Input: part model. Units: mm. Frame: model coordinates. Face numbers are marked on the shaded views. A direction names the side the tool comes from. Give positions to 0.01 mm unless a question says otherwise; leave off trailing zeros. Write each loop counter-clockwise with the first axis right and the second up, starting at its lowest first coordinate (ties: lowest second). Pieces come first, ordered by that corner, then holes. Notation, with made-up numbers: (41.5, -6) -> (54.5, -6) arc R24 cw to (54.5, 24) -> close; hole circle Ø1 at (-30.5, 35). An arc over 180 degrees is marked (long way). Answer as a JSON object with one key per item and string values. Group by question number.
from build123d import *

# Parameters (mm, degrees)
SKETCH1_R                = 6.45
BOSS_EXTRUDE1_DEPTH      = 6.35
FILLET1_R                = 2
SKETCH3_R                = 7.95
SKETCH3_R_2              = 6.45
BOSS_EXTRUDE3_DEPTH      = 3
BOSS_EXTRUDE3_DEPTH_BACK = 15.7
BOSS_EXTRUDE4_DEPTH      = 2
BOSS_EXTRUDE5_DEPTH      = 2
BOSS_EXTRUDE6_DEPTH      = 8.7


with BuildPart() as part:
    # Sketch1 → Boss-Extrude1 (new body, symmetric)
    with BuildSketch(Plane(origin=(0, 0, 0), x_dir=(1, 0, 0), z_dir=(0, 1, 0))):
        Polygon((0, -15.9), (13.76980392, 7.95), (-13.76980392, 7.95), align=None)
        with Locations(Location((0, 0, 0), (0, 0, 270))):  # turned: the seam where the file's is
            Circle(SKETCH1_R, mode=Mode.SUBTRACT)
    extrude(amount=BOSS_EXTRUDE1_DEPTH, both=True)

    # Fillet1
    fillet1_edges = [part.edges().sort_by_distance(p)[0] for p in [
        (-13.76980392, 0, -7.95),
        (13.76980392, 0, -7.95),
        (0, 0, 15.9),
    ]]
    fillet(fillet1_edges, radius=FILLET1_R)

    # Sketch3 → Boss-Extrude3 (add, two sides)
    with BuildSketch(Plane(origin=(0, 6.35, 0), x_dir=(1, 0, 0), z_dir=(0, 1, 0))) as boss_extrude3_sk:
        with Locations(Location((0, 0, 0), (0, 0, 270))):  # turned: the seam where the file's is
            Circle(SKETCH3_R)
        with Locations(Location((0, 0, 0), (0, 0, 270))):  # turned: the seam where the file's is
            Circle(SKETCH3_R_2, mode=Mode.SUBTRACT)
    extrude(amount=BOSS_EXTRUDE3_DEPTH)
    extrude(boss_extrude3_sk.sketch, amount=-BOSS_EXTRUDE3_DEPTH_BACK)

    # Sketch4 → Boss-Extrude4 (add)
    with BuildSketch(Plane(origin=(0, 6.35, 0), x_dir=(1, 0, 0), z_dir=(0, 1, 0))):
        with BuildLine():
            Line((8.183940066, -4.725), (13.336791218, 4.2))
            ThreePointArc((13.336791218, 4.2), (13.336791218, 7.7), (10.305702305, 9.45))
            Line((10.305702305, 9.45), (0, 9.45))
            Line((0, 9.45), (-10.305702305, 9.45))
            ThreePointArc((-10.305702305, 9.45), (-13.336791218, 7.7), (-13.336791218, 4.2))
            Line((-13.336791218, 4.2), (-8.183940066, -4.725))
            Line((-8.183940066, -4.725), (-3.031088913, -13.65))
            ThreePointArc((-3.031088913, -13.65), (0, -15.4), (3.031088913, -13.65))
            Line((3.031088913, -13.65), (8.183940066, -4.725))
        make_face()
        with BuildLine():
            Line((6.88490196, -3.975), (12.037753113, 4.95))
            ThreePointArc((12.037753113, 4.95), (12.037753113, 6.95), (10.305702305, 7.95))
            Line((10.305702305, 7.95), (0, 7.95))
            Line((0, 7.95), (-10.305702305, 7.95))
            ThreePointArc((-10.305702305, 7.95), (-12.037753113, 6.95), (-12.037753113, 4.95))
            Line((-12.037753113, 4.95), (-6.88490196, -3.975))
            Line((-6.88490196, -3.975), (-1.732050808, -12.9))
            ThreePointArc((-1.732050808, -12.9), (0, -13.9), (1.732050808, -12.9))
            Line((1.732050808, -12.9), (6.88490196, -3.975))
        make_face(mode=Mode.SUBTRACT)
    extrude(amount=-BOSS_EXTRUDE4_DEPTH)

    # Sketch5 → Boss-Extrude5 (add)
    with BuildSketch(Plane.XZ.offset(6.35)):
        with BuildLine():
            Line((13.336791218, -4.2), (3.031088913, 13.65))
            ThreePointArc((3.031088913, 13.65), (0, 15.4), (-3.031088913, 13.65))
            Line((-3.031088913, 13.65), (-13.336791218, -4.2))
            ThreePointArc((-13.336791218, -4.2), (-13.336791218, -7.7), (-10.305702305, -9.45))
            Line((-10.305702305, -9.45), (10.305702305, -9.45))
            ThreePointArc((10.305702305, -9.45), (13.336791218, -7.7), (13.336791218, -4.2))
        make_face()
        with BuildLine():
            Line((10.305702305, -7.95), (-10.305702305, -7.95))
            ThreePointArc((-10.305702305, -7.95), (-12.037753113, -6.95), (-12.037753113, -4.95))
            Line((-12.037753113, -4.95), (-1.732050808, 12.9))
            ThreePointArc((-1.732050808, 12.9), (0, 13.9), (1.732050808, 12.9))
            Line((1.732050808, 12.9), (12.037753113, -4.95))
            ThreePointArc((12.037753113, -4.95), (12.037753113, -6.95), (10.305702305, -7.95))
        make_face(mode=Mode.SUBTRACT)
    extrude(amount=-BOSS_EXTRUDE5_DEPTH)

    # Sketch6 → Boss-Extrude6 (add)
    with BuildSketch(Plane.XZ.offset(-4.35)):
        with BuildLine():
            Line((-2.165063509, 13.15), (-3.031088913, 13.65))
            ThreePointArc((-3.031088913, 13.65), (0, 15.4), (3.031088913, 13.65))
            Line((3.031088913, 13.65), (2.165063509, 13.15))
            ThreePointArc((2.165063509, 13.15), (1.864007283, 13.565976245), (1.484313483, 13.911669328))
            Line((1.484313483, 13.911669328), (1, 13.632050808))
            ThreePointArc((1, 13.632050808), (0, 13.9), (-1, 13.632050808))
            Line((-1, 13.632050808), (-1.484313483, 13.911669328))
            ThreePointArc((-1.484313483, 13.911669328), (-1.864007283, 13.565976245), (-2.165063509, 13.15))
        make_face()
    extrude(amount=BOSS_EXTRUDE6_DEPTH)


solid = part.part
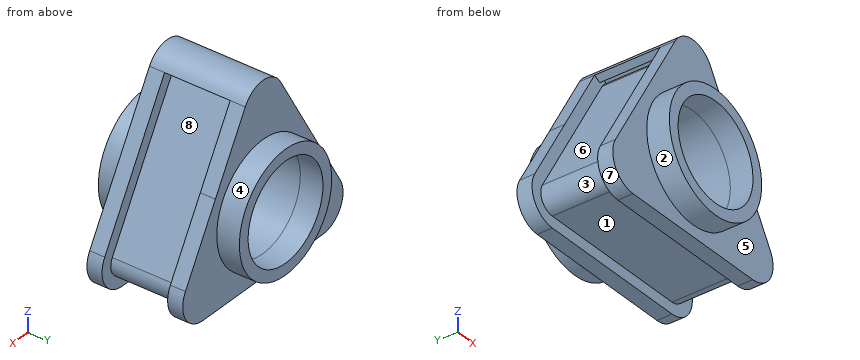
1. Section B-B (y = -2.5). Return the cut outline in (x, z), plus the area to 3 significant figures.
2. Section A-A (x = 0). Return the cut outline in (y, z), plus the area to 3 significant figures.
3. Section C-C (z = 0). Return the cut outline in (x, y).
4. Line query: line 1 (X direction, y = 7.4, z = 0); line 2 (Y direction, x = 12.5, z = -6.75); line 3 (Z direction, x = -1.25, y = 0.25). Output: solid intervals per line, ascending.
5. Section D-D (z = 6). Return the cut outline in (x, y), plus the area to 3 significant figures.
6. Mould query, pull axis Y, two halves, no side actions, for the marked faces 5, 6, 7 and 8. Classes: pulls with the +Y half, pulls with the -Y half, needs draft (parallel to the pull), parting line crosses it, or undercut.
7. Contact query for flat-ended pins moving along their axis: pin 1 Ø1.5 at (x, y) = (9.5, 0.5) entering from +Z; pin 2 Ø2 at (x, y) = (-4, 1) entering from +Z; pin 3 Ø6 at (x, y) = (1.5, -0.5) entering from -Z. Output: stop coordinate, or through.
8. Reachability of the marked faces 1, 2, 3 and 4 from +Z, -Z, +X, -X, +Y, -Y: full face, straight path, thin tool, end or side. Return the list, or none.
Working result:
{
 "1": {"outline": "(-12.04, -4.95) arc R2 ccw to (-10.31, -7.95) -> (10.31, -7.95) arc R2 ccw to (12.04, -4.95) -> (1.73, 12.9) arc R2 ccw to (1, 13.63) -> (1.48, 13.91) arc R2.5 cw to (2.17, 13.15) -> (3.03, 13.65) arc R3.5 ccw to (-3.03, 13.65) -> (-2.17, 13.15) arc R2.5 cw to (-1.48, 13.91) -> (-1, 13.63) arc R2 ccw to (-1.73, 12.9) -> close; hole circle Ø12.9 at (0, 0)", "area": "197 mm^2"},
 "2": {"outline": "(-9.35, -7.95) -> (-6.35, -7.95) -> (-6.35, -9.45) -> (-4.35, -9.45) -> (-4.35, -7.95) -> (4.35, -7.95) -> (4.35, -9.45) -> (6.35, -9.45) -> (6.35, -7.95) -> (9.35, -7.95) -> (9.35, -6.45) -> (-9.35, -6.45) -> close; (-9.35, 6.45) -> (9.35, 6.45) -> (9.35, 7.95) -> (6.35, 7.95) -> (6.35, 15.4) -> (-6.35, 15.4) -> (-6.35, 7.95) -> (-9.35, 7.95) -> close", "area": "157 mm^2"},
 "3": {"outline": "(-10.91, -6.35) -> (-7.95, -6.35) -> (-7.95, -9.35) -> (-6.45, -9.35) -> (-6.45, 9.35) -> (-7.95, 9.35) -> (-7.95, 6.35) -> (-10.91, 6.35) -> (-10.91, 4.35) -> (-9.18, 4.35) -> (-9.18, -4.35) -> (-10.91, -4.35) -> close; (6.45, -9.35) -> (7.95, -9.35) -> (7.95, -6.35) -> (10.91, -6.35) -> (10.91, -4.35) -> (9.18, -4.35) -> (9.18, 4.35) -> (10.91, 4.35) -> (10.91, 6.35) -> (7.95, 6.35) -> (7.95, 9.35) -> (6.45, 9.35) -> close"},
 "4": {"line 1": "x = -7.95 to -6.45, 6.45 to 7.95", "line 2": "y = -6.35 to -4.35, 4.35 to 6.35", "line 3": "z = -7.95 to -6.33, 6.33 to 13.46, 13.78 to 15.17"},
 "5": {"outline": "(-7.45, -6.35) -> (-5.22, -6.35) -> (-5.22, -9.35) -> (-2.37, -9.35) -> (-2.37, 9.35) -> (-5.22, 9.35) -> (-5.22, 6.35) -> (-7.45, 6.35) -> (-7.45, 4.35) -> (-5.72, 4.35) -> (-5.72, -4.35) -> (-7.45, -4.35) -> close; (2.37, -9.35) -> (5.22, -9.35) -> (5.22, -6.35) -> (7.45, -6.35) -> (7.45, -4.35) -> (5.72, -4.35) -> (5.72, 4.35) -> (7.45, 4.35) -> (7.45, 6.35) -> (5.22, 6.35) -> (5.22, 9.35) -> (2.37, 9.35) -> close", "area": "133 mm^2"},
 "6": {"face 5": "pulls with the -Y half", "face 6": "undercut", "face 7": "needs draft", "face 8": "undercut"},
 "7": {"pin 1": "stops at z = 0.74", "pin 2": "stops at z = 13.7", "pin 3": "stops at z = -7.95"},
 "8": {"face 1": "-Z, +X, -X", "face 2": "-Y", "face 3": "-X", "face 4": "+Y"}
}
